Input: part model. Units: mm. Frame: model coordinates. A direction names the side the tool comes from. Round coordinates to 2 decimals unless told otherwise and drop trailing zeros. Put each result on its own line as item: value. Start each with the question number.
1) Line query: probe 1 along Y at (x, z) = (-2.5, 19.5); probe 2 along X at (y, z) = (6, 2.75); probe 3 along X at (y, z) = (4, 15.25). Output: solid intervals per line, ascending.
2) Reachability of faces 3 (the face through (-1, -55, 25.4)), 4 (the face through (-25.324, -36.679, 22.896)) from +Z, -Z, +X, -X, +Y, -Y: full face, straight path, thin tool, end or side. Return the list, or none.
3) Pin query (flat end, axial travel): pin 1 (12 mm diameter, centred on x = -13, y = -21.5, fed in from +Z); pin 2 (5 mm diameter, centred on y = 9.5, z = 17.5, fed in from -X); pin 3 (1 mm diameter, centred on x = -24, z = 5, fed in from -Y); pin 4 (12 mm diameter, centred on y = 10, z = 17.5, fed in from +X). Return the tip coordinate at first contact, or that it passes through.
4) Draft query along X for faces 1 (the face through (13.38, 0.09, 22.45)), 2 (the face through (3, -49, 0)). Return one class per face: +X half, -X half, draft (parallel to the pull), parting line (faces both ways), or undercut.
from build123d import *

# Parameters (mm, degrees)
F1_DEPTH     = 25.4
F3_DEPTH     = 50.8
F5_T4_DEPTH  = 64.0057067986
F5_T9_DEPTH  = 86.9283653755
F5_T15_DEPTH = 60.9737188004
F5_T20_DEPTH = 59.1061688919
F5_T25_DEPTH = 43.6640606018
F5_T31_DEPTH = 57.4502846001


# Not quite as in the source:
# - a fillet or chamfer that OpenCascade refuses, or shapes differently, is made with other operations: its cross-section is extruded or revolved along the edge and cut away or added
# - a feature of the source that left no trace in its solid (it failed there, or was rolled back) is left out


with BuildPart() as f1:
    # F0 (on Top) → F1 (new body)
    with BuildSketch(Plane.XY):
        with BuildLine():
            add(Edge.make_bspline(
                [(-48.315115273, -59.7526505589), (-37.5784229901, -46.4742837681), (-26.8417307072, -33.1959169772), (-16.1050384243, -19.9175501863)],
                knots=[0, 0, 0, 0, 51.2281589782, 51.2281589782, 51.2281589782, 51.2281589782], degree=3))
            add(Edge.make_bspline(
                [(-48.315115273, -59.7526505589), (-1.0274761031, -59.7958142001), (46.2601630669, -59.8389778412), (46.3316738605, -59.1182820499)],
                knots=[0, 0, 0, 0, 0.8911107377, 0.8911107377, 0.8911107377, 0.8911107377], degree=3))
            add(Edge.make_bspline(
                [(46.3316738605, -59.1182820499), (46.3235373894, -59.1079000767), (46.3154009182, -59.0975181035), (46.3072644471, -59.0871361303)],
                knots=[0, 0, 0, 0, 0.0395712999, 0.0395712999, 0.0395712999, 0.0395712999], degree=3))
            add(Edge.make_bspline(
                [(46.3072644471, -59.0871361303), (36.0194733937, -45.9601220924), (25.7316823403, -32.8331080545), (15.4438912868, -19.7060940166)],
                knots=[0.0395712999, 0.0395712999, 0.0395712999, 0.0395712999, 50.0737024584, 50.0737024584, 50.0737024584, 50.0737024584], degree=3))
            add(Edge.make_bspline(
                [(15.4438912868, -19.7060940166), (10.2959275246, -13.1373960111), (5.1479637623, -6.5686980055), (0, 0)],
                knots=[50.0737024584, 50.0737024584, 50.0737024584, 50.0737024584, 75.1105536876, 75.1105536876, 75.1105536876, 75.1105536876], degree=3))
            add(Edge.make_bspline(
                [(-16.1050384243, -19.9175501863), (-10.7366922829, -13.2783667909), (-5.3683461414, -6.6391833954), (0, 0)],
                knots=[51.2281589782, 51.2281589782, 51.2281589782, 51.2281589782, 76.8422384673, 76.8422384673, 76.8422384673, 76.8422384673], degree=3))
        make_face()
        with BuildLine():
            add(Edge.make_bspline(
                [(-16.1050384243, -19.9175501863), (-15.0708617229, -7.3149574714), (-14.0366850214, 5.2876352436), (-13.0025083199, 17.8902279586)],
                knots=[0, 0, 0, 0, 37.9348623472, 37.9348623472, 37.9348623472, 37.9348623472], degree=3))
            add(Edge.make_bspline(
                [(-16.1050384243, -19.9175501863), (-10.7366922829, -13.2783667909), (-5.3683461414, -6.6391833954), (0, 0)],
                knots=[51.2281589782, 51.2281589782, 51.2281589782, 51.2281589782, 76.8422384673, 76.8422384673, 76.8422384673, 76.8422384673], degree=3))
            add(Edge.make_bspline(
                [(15.4438912868, -19.7060940166), (10.2959275246, -13.1373960111), (5.1479637623, -6.5686980055), (0, 0)],
                knots=[50.0737024584, 50.0737024584, 50.0737024584, 50.0737024584, 75.1105536876, 75.1105536876, 75.1105536876, 75.1105536876], degree=3))
            add(Edge.make_bspline(
                [(15.4438912868, -19.7060940166), (15.4438912868, -6.5000866436), (15.4438912868, 6.7059207294), (15.4438912868, 19.9119281024)],
                knots=[0, 0, 0, 0, 39.618022119, 39.618022119, 39.618022119, 39.618022119], degree=3))
            add(Edge.make_bspline(
                [(15.4438912868, 19.9119281024), (5.9617580846, 19.2380280544), (-3.5203751177, 18.5641280065), (-13.0025083199, 17.8902279586)],
                knots=[0, 0, 0, 0, 28.5181507475, 28.5181507475, 28.5181507475, 28.5181507475], degree=3))
        make_face()
    extrude(amount=F1_DEPTH)

    # F2 (on Top) → F3 (cut)
    with BuildSketch(Plane.XY):
        with BuildLine():
            add(Edge.make_bspline(
                [(11.2517978996, 14.0004176646), (5.4347412661, 13.426968207), (-0.3823153675, 12.8535187493), (-6.199372001, 12.2800692916)],
                knots=[0, 0, 0, 0, 17.5357614441, 17.5357614441, 17.5357614441, 17.5357614441], degree=3))
            add(Edge.make_bspline(
                [(-6.199372001, 12.2800692916), (-6.8688768273, 1.8608955046), (-7.5383816535, -8.5582782825), (-8.2078864798, -18.9774520695)],
                knots=[0, 0, 0, 0, 31.3219854424, 31.3219854424, 31.3219854424, 31.3219854424], degree=3))
            add(Edge.make_bspline(
                [(-8.2078864798, -18.9774520695), (-15.9868902216, -28.9221989612), (-23.7658939635, -38.8669458528), (-31.5448977053, -48.8116927445)],
                knots=[0, 0, 0, 0, 37.8774076409, 37.8774076409, 37.8774076409, 37.8774076409], degree=3))
            add(Edge.make_bspline(
                [(-31.5448977053, -48.8116927445), (-14.2238239447, -48.8116927445), (3.0972498159, -48.8116927445), (20.4183235765, -48.8116927445)],
                knots=[0, 0, 0, 0, 51.9632212818, 51.9632212818, 51.9632212818, 51.9632212818], degree=3))
            add(Edge.make_bspline(
                [(20.4183235765, -48.8116927445), (23.3639385551, -48.8116927445), (26.3095535338, -48.8116927445), (29.2551685125, -48.8116927445)],
                knots=[0, 0, 0, 0, 8.836844936, 8.836844936, 8.836844936, 8.836844936], degree=3))
            add(Edge.make_bspline(
                [(29.2551685125, -48.8116927445), (23.2540449748, -38.8669458528), (17.2529214372, -28.9221989612), (11.2517978996, -18.9774520695)],
                knots=[0, 0, 0, 0, 34.8454196427, 34.8454196427, 34.8454196427, 34.8454196427], degree=3))
            add(Edge.make_bspline(
                [(11.2517978996, -18.9774520695), (11.2517978996, -7.9848288248), (11.2517978996, 3.0077944199), (11.2517978996, 14.0004176646)],
                knots=[0, 0, 0, 0, 32.9778697342, 32.9778697342, 32.9778697342, 32.9778697342], degree=3))
        make_face()
    extrude(amount=F3_DEPTH, mode=Mode.SUBTRACT)

    # F5: chamfer of 5.08 on 6 edges, made by hand


with BuildPart() as f5_tool2:
    # F5_s3 → F5_t4 (new body)
    with BuildSketch(Plane(origin=(-43.7113633895, -55.8809919142, 0), x_dir=(0, 0, 1), z_dir=(0.6161195467, 0.7876526545, 0))):
        Polygon((25.4, 0.1474155925), (20.32, 5.2274155925), (25.4, 5.2274155925), align=None)
    extrude(amount=F5_T4_DEPTH)

    split(bisect_by=Plane(origin=(0, -14.2458463722, -14.2458463722), x_dir=(1, 0, 0), z_dir=(0, 0.7071067812, 0.7071067812)), keep=Keep.TOP)


with BuildPart() as f1_1:
    add(f1.part)

    # F5_t1: cut F5_tool2
    add(f5_tool2.part, mode=Mode.SUBTRACT)


with BuildPart() as f5_tool7:
    # F5_s8 → F5_t9 (new body)
    with BuildSketch(Plane.YZ.offset(-44.6090472842)):
        Polygon((-53.8916927445, 25.4), (-48.8116927445, 20.32), (-48.8116927445, 25.4), align=None)
    extrude(amount=F5_T9_DEPTH)

    split(bisect_by=Plane(origin=(-8.7722085747, -5.293559296, 10.2456533856), x_dir=(0.5166639058, -0.856188302, 0), z_dir=(-0.6054165543, -0.3653365514, 0.7071067812)), keep=Keep.TOP)

    split(bisect_by=Plane(origin=(10.0612448539, -7.870131057, 12.7737077963), x_dir=(0.6161195467, 0.7876526545, 0), z_dir=(0.5569545332, -0.4356623095, 0.7071067812)), keep=Keep.TOP)


with BuildPart() as f1_2:
    add(f1_1.part)

    # F5_t6: cut F5_tool7
    add(f5_tool7.part, mode=Mode.SUBTRACT)


with BuildPart() as f5_tool13:
    # F5_s14 → F5_t15 (new body)
    with BuildSketch(Plane(origin=(4.6486942055, -7.7035719995, 0), x_dir=(0, 0, 1), z_dir=(0.5166639058, -0.856188302, 0))):
        Polygon((25.4, -4.9086932287), (20.32, 0.1713067713), (25.4, 0.1713067713), align=None)
    extrude(amount=F5_T15_DEPTH)

    split(bisect_by=Plane(origin=(0, -14.2458463722, -14.2458463722), x_dir=(1, 0, 0), z_dir=(0, 0.7071067812, 0.7071067812)), keep=Keep.TOP)


with BuildPart() as f1_3:
    add(f1_2.part)

    # F5_t12: cut F5_tool13
    add(f5_tool13.part, mode=Mode.SUBTRACT)


with BuildPart() as f5_tool18:
    # F5_s19 → F5_t20 (new body)
    with BuildSketch(Plane.XZ.offset(-27.0645672435)):
        Polygon((16.3317978996, 25.4), (11.2517978996, 20.32), (11.2517978996, 25.4), align=None)
    extrude(amount=F5_T20_DEPTH)

    split(bisect_by=Plane(origin=(0.3674517714, -3.7274213716, 3.7454894054), x_dir=(0.9951760553, 0.0981051424, 0), z_dir=(0.0693708114, -0.7036957372, 0.7071067812)), keep=Keep.TOP)


with BuildPart() as f1_4:
    add(f1_3.part)

    # F5_t17: cut F5_tool18
    add(f5_tool18.part, mode=Mode.SUBTRACT)


with BuildPart() as f5_tool23:
    # F5_s24 → F5_t25 (new body)
    with BuildSketch(Plane(origin=(-17.9419078945, -1.7687256632, 0), x_dir=(0, 0, 1), z_dir=(0.9951760553, 0.0981051424, 0))):
        Polygon((25.4, -17.9090211892), (20.32, -12.8290211892), (25.4, -12.8290211892), align=None)
    extrude(amount=F5_T25_DEPTH)

    split(bisect_by=Plane(origin=(6.6592316135, -0.4279022306, 6.672965308), x_dir=(0.0641247498, 0.9979418903, 0), z_dir=(0.7056514779, -0.0453430454, 0.7071067812)), keep=Keep.TOP)

    split(bisect_by=Plane(origin=(-4.5341010502, 0, 4.5341010502), x_dir=(0, 1, 0), z_dir=(-0.7071067812, 0, 0.7071067812)), keep=Keep.TOP)


with BuildPart() as f1_5:
    add(f1_4.part)

    # F5_t22: cut F5_tool23
    add(f5_tool23.part, mode=Mode.SUBTRACT)


with BuildPart() as f5_tool29:
    # F5_s30 → F5_t31 (new body)
    with BuildSketch(Plane(origin=(-2.0859058182, -32.4619246499, 0), x_dir=(0, 0, 1), z_dir=(0.0641247498, 0.9979418903, 0))):
        Polygon((25.4, -12.054069384), (20.32, -6.974069384), (25.4, -6.974069384), align=None)
    extrude(amount=F5_T31_DEPTH)

    split(bisect_by=Plane(origin=(0.3674517714, -3.7274213716, 3.7454894054), x_dir=(0.9951760553, 0.0981051424, 0), z_dir=(0.0693708114, -0.7036957372, 0.7071067812)), keep=Keep.TOP)


with BuildPart() as f1_6:
    add(f1_5.part)

    # F5_t28: cut F5_tool29
    add(f5_tool29.part, mode=Mode.SUBTRACT)


solid = f1_6.part
Geometry results:
1. probe 1: y = -59.77 to -48.81, 12.64 to 18.64
1. probe 2: x = -13.98 to -6.6, 11.25 to 15.44
1. probe 3: x = -14.14 to -6.73, 11.25 to 15.44
2. face 3: +Z, +X, -X, +Y, -Y
2. face 4: +Z
3. pin 1: stops at z = 25.4
3. pin 2: stops at x = -13.9
3. pin 3: stops at y = -59.77
3. pin 4: stops at x = 15.44
4. face 1: undercut
4. face 2: draft
